Input: part model. Units: mm. Frame: model coordinates. A direction names the side the tool comes from. Coordinates: 2 decimals unless noted, no trailing zeros. Write each loop counter-clockwise with the first axis right and the second up, starting at its lowest first coordinate (ties: lowest second). Pieces come first, ordered by that corner, then holes. Notation, with made-up numbers: (14, 70.5) - (48, 70.5) arc R27 cw to (48, 102.5) - close; hole circle Ø8 at (25, 57). An arc over 180 degrees is marked (long way). Use CSV: the item, a comma, the result in double quotes.
Autodesk Inventor part; units mm, degrees
ref_plane "YZ Plane" through (0, 0, 0) normal (1, 0, 0) x (0, 1, 0)
ref_plane "XZ Plane" through (0, 0, 0) normal (0, 1, 0) x (-1, 0, 0)
ref_plane "XY Plane" through (0, 0, 0) normal (0, 0, 1) x (1, 0, 0)
sketch "Sketch1" plane through (0, 0, 0) normal (0, 0, 1) x (1, 0, 0)
  circle A0 centre (0, 0) radius 40
  circle A1 centre (0, 0) radius 49.975
  dimension "d0" = 80
  dimension "d1" = 99.95
extrude "Extrusion1" add sketch "Sketch1" along normal blind 10
sketch "Sketch2" plane through (0, 0, 10) normal (0, 0, 1) x (1, 0, 0)
  circle A0 centre (0, 0) radius 49.975
  circle A1 centre (0, 0) radius 40
  circle A2 centre (0, 0) radius 48.475
  circle A3 centre (0, 0) radius 42
  dimension "d4" = 1.5
  dimension "d5" = 2
extrude "Extrusion2" cut sketch "Sketch2" against normal blind 0.5 contours A2
sketch "Sketch3" plane through (0, 0, 0) normal (0, 0, -1) x (-1, 0, 0)
  circle A0 centre (0, 0) radius 42
  circle A1 centre (0, 0) radius 48.475
extrude "Extrusion3" cut sketch "Sketch3" against normal blind 0.5
properties part number "bearing_100x80x10"
(1) Reachability of faces 4 (the cylindrical face through (-22.368, -43.006, 0.246)), 5 (the flat face through (-15, 40, 9.5)), 6 (the flat face through (37.1, -15.4, 0)) from +Z, -Z, +X, -X, +Y, -Y: full face, straight path, thin tool, end or side. Return the list, or none.
Check values:
face 4,"-Z"
face 5,"+Z"
face 6,"-Z, +X, -X, +Y, -Y"
(2) Draft query along Y for faces 1 (the flat face through (15, 40, 0.5)), 2 (the flat face through (-8, 48, 0)), 3 (the cylindrical face through (-39.66, 30.41, 4.93)). Return one class per face: pulls with the +Y half, pulls with the -Y half, needs draft (parallel to the pull), parting line crosses it, or undercut.
Check values:
face 1,"undercut"
face 2,"needs draft"
face 3,"parting line crosses it"
(3) Cut plane A-A on x = 0. Return loops of the section in (y, z) (3 decimals).
Check values:
outline,"(-49.975, 0) - (-48.475, 0) - (-48.475, 0.5) - (-42, 0.5) - (-42, 0) - (-40, 0) - (-40, 10) - (-42, 10) - (-42, 9.5) - (-48.475, 9.5) - (-48.475, 10) - (-49.975, 10) - close; (40, 0) - (42, 0) - (42, 0.5) - (48.475, 0.5) - (48.475, 0) - (49.975, 0) - (49.975, 10) - (48.475, 10) - (48.475, 9.5) - (42, 9.5) - (42, 10) - (40, 10) - close"
(4) Ray query, probe 1 along Y at (x, z) = (0, 0.4) (3 decimals); probe 2 along Y at (x, z) = (0, 4.5) (3 decimals); probe 3 along X at (y, z) = (-22, 9). Return the intervals inside material, ascending. Write a range as from..to.
Check values:
probe 1,"-49.975..-48.475, -42..-40, 40..42, 48.475..49.975"
probe 2,"-49.975..-40, 40..49.975"
probe 3,"-44.87..-33.41, 33.41..44.87"
(5) Pin query (flat end, axial travel): pin 1 Ø1 at (x, z) = (29, 4) entering from -Y; pin 2 Ø3 at (y, z) = (15, 6.5) entering from -X; pin 3 Ø5 at (y, z) = (24.5, 5) entering from -X. Return the tip coordinate at first contact, or that it passes through.
Check values:
pin 1,"y = -41.05"
pin 2,"x = -48.12"
pin 3,"x = -44.87"
(6) Cut plane C-C on z = 6.25. Return loops of the section in (x, y) (3 decimals).
Check values:
outline,"circle Ø99.95 at (0, 0); hole circle Ø80 at (0, 0)"
